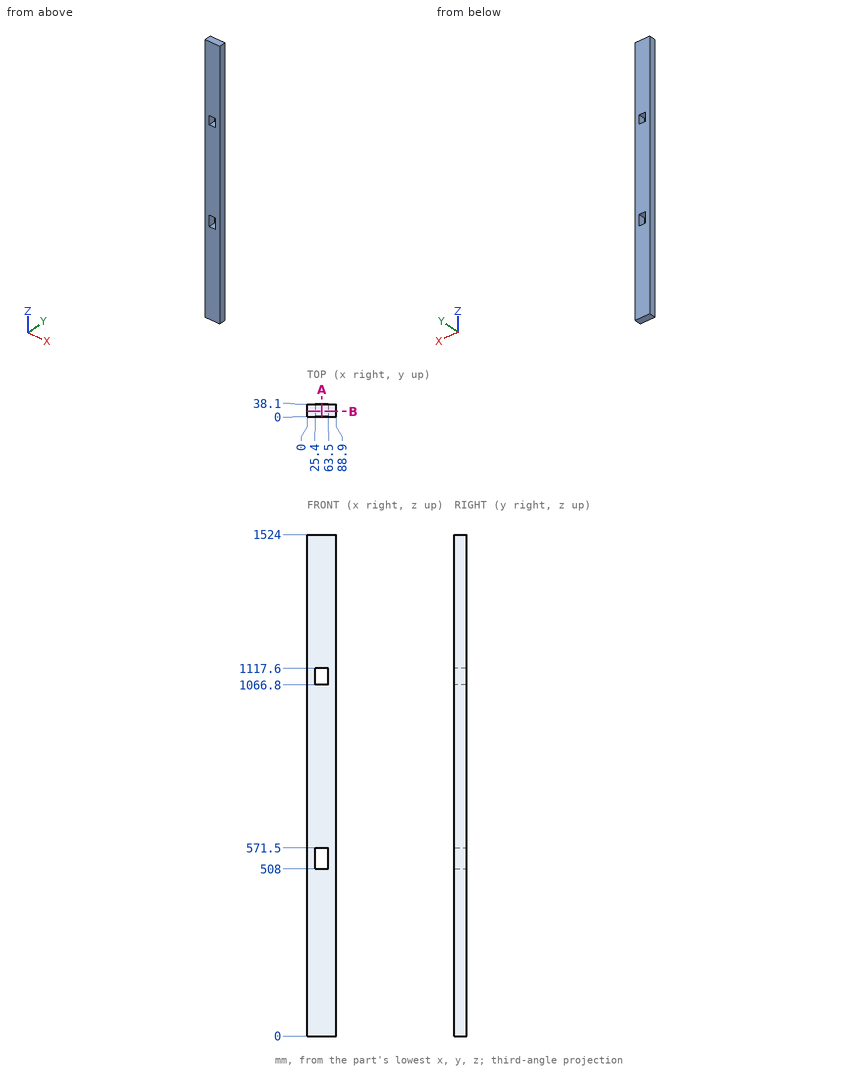
Here's the drawing with two shaded views (mm, measured from the low corner). I have some questions. Coordinates: 2 decimals unless noted, no trailing zeros. Order: outer loops, then holes, each group sorted by start corner. A loop starts at its lowest first (then second) coordinate and runs counter-clockwise, first axis right, second up.
Item 1: If we section it at A-A, the plane x = 44.5: List the corners of the cut face in (y, z) for me, then the cut area to 3 significant figures.
Response values:
outline: (0, 0) - (38.1, 0) - (38.1, 508) - (0, 508) - close; (0, 571.5) - (38.1, 571.5) - (38.1, 1066.8) - (0, 1066.8) - close; (0, 1117.6) - (38.1, 1117.6) - (38.1, 1524) - (0, 1524) - close
area: 53,700 mm2
Item 2: If we section it at B-B, the plane y = 16: List the corners of the cut face in (x, z) for me.
Response values:
outline: (0, 0) - (88.9, 0) - (88.9, 1524) - (0, 1524) - close; hole (25.4, 508) - (63.5, 508) - (63.5, 571.5) - (25.4, 571.5) - close; hole (25.4, 1066.8) - (63.5, 1066.8) - (63.5, 1117.6) - (25.4, 1117.6) - close
Item 3: I need wall thicknesses on probe 1 along Z at (x, y) = (35.5, 19); probe 2 along X at (y, z) = (3, 1072.5). Which ranges of each line are inside material? Lowest first, please.
Response values:
probe 1: z = 0 to 508, 571.5 to 1066.8, 1117.6 to 1524
probe 2: x = 0 to 25.4, 63.5 to 88.9
Item 4: I'm going to push a flat-ended pin straight in: pin 1 Ø8 at (x, z) = (32.5, 551.5) entering from +Y. Where does the tip first touch, or does it pass through?
Response values:
pin 1: passes through
